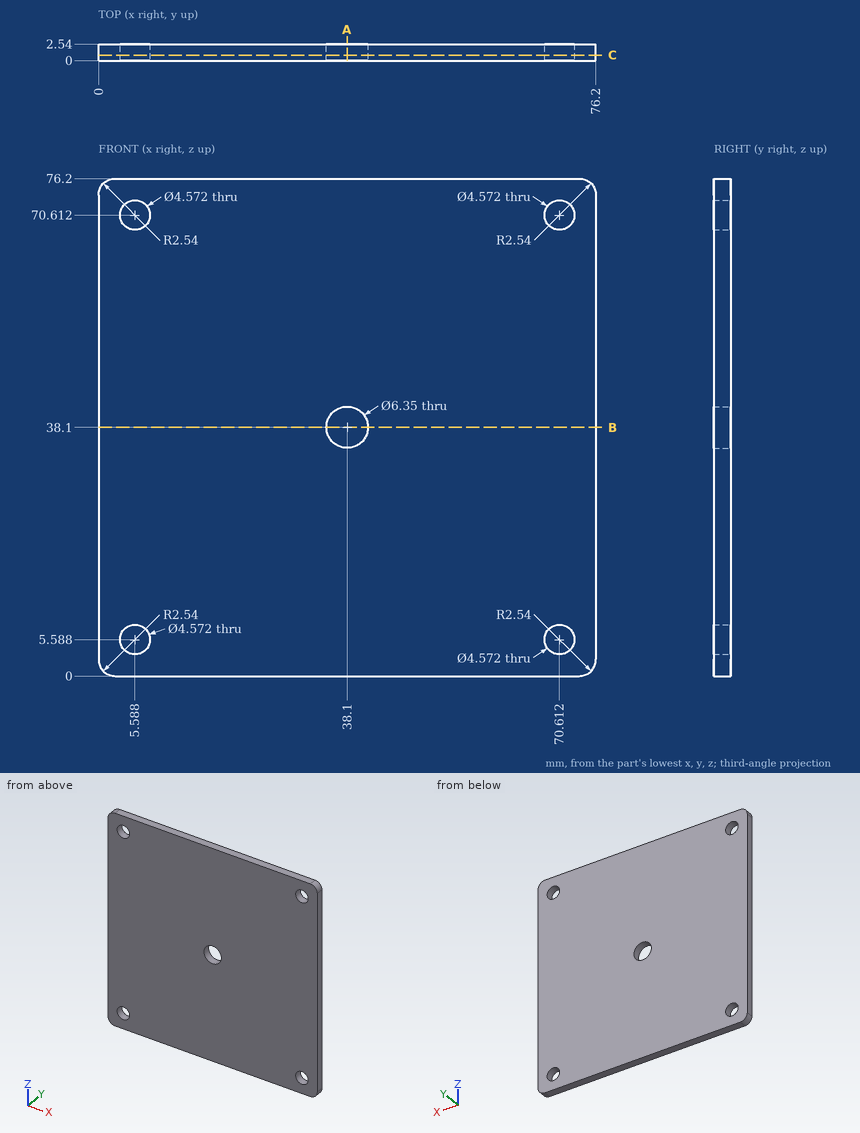
Check sheet for the drawn part. Datum: minimum x, y, z corner. Units: mm. Give positions to 0.01 mm unless a question says otherwise; leave off trailing zeros. Loops run counter-clockwise (first coordinate to the right, second up) from the corner with the lowest first, then second, coordinate; pieces in that order, holes last. Notation, with made-up numbers: M -33.5,36.5 L -26.5,36.5 A28 ccw -26.5,54.5 Z; hole C -39,75 d6. An arc over 180 degrees is marked long. Answer as CSV lines item,"result".
Item 1: Sectioned sample at C-C, the plane y = 0.85. Enter the section's corners in (x, z) (3 decimals), then the cut area to 3 significant figures.
Reply:
outline,"M 0,2.54 A2.54 ccw 2.54,0 L 73.66,0 A2.54 ccw 76.2,2.54 L 76.2,73.66 A2.54 ccw 73.66,76.2 L 2.54,76.2 A2.54 ccw 0,73.66 Z; hole C 5.588,5.588 d4.572; hole C 5.588,70.612 d4.572; hole C 38.1,38.1 d6.35; hole C 70.612,5.588 d4.572; hole C 70.612,70.612 d4.572"
area,"5,700 mm^2"
Item 2: Sectioned sample at A-A, the plane x = 38.1. Enter the section's corners in (y, z) (3 decimals), then the cut area to 3 significant figures.
Reply:
outline,"M 0,0 L 2.54,0 L 2.54,34.925 L 0,34.925 Z; M 0,41.275 L 2.54,41.275 L 2.54,76.2 L 0,76.2 Z"
area,"177 mm^2"
Item 3: Sectioned sample at B-B, the plane z = 38.1. Enter the section's corners in (x, y) (3 decimals).
Reply:
outline,"M 0,0 L 34.925,0 L 34.925,2.54 L 0,2.54 Z; M 41.275,0 L 76.2,0 L 76.2,2.54 L 41.275,2.54 Z"
Item 4: Scan lines: L1, parallel to X at y = 0.85, z = 38.1 (3 decimals); L2, parallel to Z at x = 7.5, y = 1.15; L3, parallel to X at y = 0.65, z = 69. Record each from-to range of solid material in increasing order.
Reply:
L1,"0 to 34.925, 41.275 to 76.2"
L2,"0 to 4.33, 6.84 to 69.36, 71.87 to 76.2"
L3,"0 to 3.97, 7.21 to 68.99, 72.23 to 76.2"
Item 5: Depth check by flat-ended pin: pin 1 Ø3.5 at (x, z) = (5.588, 70.612) entering from +Y. Enter the tip coordinate at first touch or a pass-through.
Reply:
pin 1,"through"
